Here's how the part is built. I have some questions about the finished solid (model axes, mm). Face numbers are marked on the shaded views. Give positions to 0.01 mm unless a question says otherwise; leave off trailing zeros. Write each loop counter-clockwise with the first axis right and the second up, starting at its lowest first coordinate (ties: lowest second). Pieces come first, ordered by that corner, then holes. Notation, with made-up numbers: (41.5, 31.25) - (48.5, 31.25) arc R30 cw to (48.5, 57.25) - close; hole circle Ø11 at (47, -18.5). An arc over 180 degrees is marked (long way). Use a Markdown table: item, result.
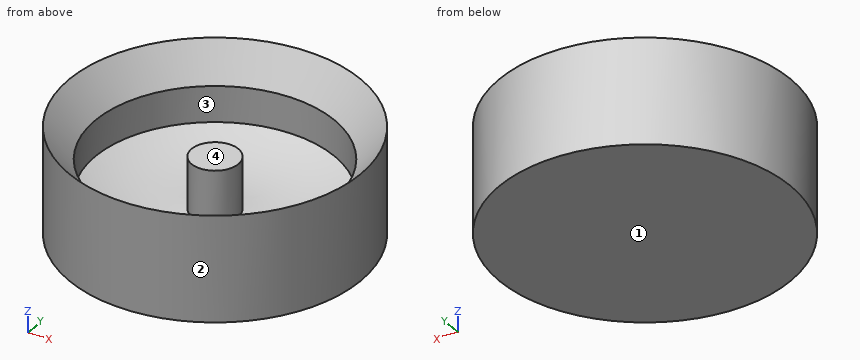
```python
from build123d import *


with BuildPart() as f1:
    # F0 (on Front) → F1 (revolve)
    with BuildSketch(Plane.XZ):
        with BuildLine():
            Line((-48.207466, 12.51955), (-48.207466, 0))
            Line((-48.207466, 0), (0, 0))
            Line((0, 0), (0, 9.353687))
            Line((0, 9.353687), (0, 25.185656))
            Line((0, 25.185656), (-7.73931, 25.185656))
            Line((-7.73931, 25.185656), (-7.73931, 8.055973))
            ThreePointArc((-7.73931, 8.055973), (-23.932162, 8.32034), (-39.573293, 12.51955))
            Line((-39.573293, 12.51955), (-39.573293, 24.319587))
            Line((-39.573293, 24.319587), (-48.207466, 34.968402))
            Line((-48.207466, 34.968402), (-48.207466, 24.319587))
            Line((-48.207466, 24.319587), (-48.207466, 12.51955))
        make_face()
    revolve(axis=Axis((0, 0, 17.269671), (0, 0, -1)))


solid = f1.part
```
Item 1: Will these pins go through, and if not, where does the flat tip stop? pin 1 Ø3 at (x, z) = (-26, 11) entering from -Y; pin 2 Ø5 at (x, z) = (-36.5, 13) entering from -Y; pin 3 Ø4 at (x, z) = (26.5, 19) entering from +Y.
Values:
| item | result |
|---|---|
| pin 1 | stops at y = -41.52 |
| pin 2 | stops at y = -34.18 |
| pin 3 | stops at y = 41.52 |
Item 2: Thinking about a two-plate mould opening in Y: for the marked faces 1, 2, 3 and 4, which applies, +Y half, -Y half, draft (parallel to the pull), parting line (faces both ways), or undercut?
Values:
| item | result |
|---|---|
| face 1 | draft |
| face 2 | parting line |
| face 3 | undercut |
| face 4 | undercut |
Item 3: I need wall thicknesses on line 1 along Y through (x, z) = (0, 19); line 2 along Z through (x, y) = (11.5, 6.5); line 3 along Y through (x, z) = (2, 24). Which ranges of each line are inside material? Lowest first, please. Write a range as [from, to].
Values:
| item | result |
|---|---|
| line 1 | y = [-48.21, -39.57], [-7.74, 7.74], [39.57, 48.21] |
| line 2 | z = [0, 7.7] |
| line 3 | y = [-48.17, -39.52], [-7.48, 7.48], [39.52, 48.17] |
Item 4: If we section it at A-A, the plane z = 20: Write out the boundary of the cut face in (x, y).
Values:
| item | result |
|---|---|
| outline | circle Ø96.41 at (0, 0); circle Ø15.48 at (0, 0); hole circle Ø79.15 at (0, 0) |
